from build123d import *

# Parameters (mm, degrees)
SKETCH_R          = 2.5
PAD_DEPTH         = 30
SKETCH001_R       = 4
PAD001_DEPTH      = 3
SKETCH002_R       = 1.5
POCKET_DEPTH      = 4.001
POCKET_DEPTH_BACK = -4.001


with BuildPart() as part:
    # Sketch → Pad (new body)
    with BuildSketch(Plane.XY):
        Circle(SKETCH_R)
    extrude(amount=PAD_DEPTH)

    # Sketch001 → Pad001 (join)
    with BuildSketch(Plane.XY):
        Circle(SKETCH001_R)
    extrude(amount=PAD001_DEPTH)

    # Sketch002 → Pocket (cut, two sides)
    with BuildSketch(Plane.XZ) as pocket_sk:
        with Locations((0, 27)):
            Circle(SKETCH002_R)
    extrude(amount=-POCKET_DEPTH, mode=Mode.SUBTRACT)
    extrude(pocket_sk.sketch, amount=-POCKET_DEPTH_BACK, mode=Mode.SUBTRACT)


solid = part.part
Here's how the part is built. I have some questions about the finished solid (model axes, mm). A direction names the side the tool comes from. Round coordinates to 2 decimals unless told otherwise and drop trailing zeros. Order: outer loops, then holes, each group sorted by start corner. A loop starts at its lowest first (then second) coordinate and runs counter-clockwise, first axis right, second up. Notation, with made-up numbers: (69.25, -16.5) -> (108.25, -16.5) arc R10 cw to (108.25, -2.5) -> close; hole circle Ø4 at (25, 19.25). An arc over 180 degrees is marked (long way). Return JSON: item names as keys, results as strings.
Q1. Which directions (+Z, -Z, +X, -X, +Y, -Y) give clear straight access to the entire face, cutting with the end or side of a thin tool? Please do faces 1 (the cylindrical face through (2.385, 0.751, 16.311)), 2 (the flat face through (0, 0, 30)).
Filled sheet:
{"face 1": "+Z", "face 2": "+Z, +X, -X, +Y, -Y"}
Q2. If we mould it in two halves opening along Z, with no side actions, what happens to faces 3 (the flat face through (0, 0, 0)), 4 (the cylindrical face through (-0.867, -3.905, 1.479)), 5 (the cylindrical face through (-1.5, -0.04, 27.07)), 6 (the flat face through (2, 2, 3))? For each: released by +Z, released by -Z, zero draft, split by the parting line, or undercut.
Filled sheet:
{"face 3": "released by -Z", "face 4": "zero draft", "face 5": "undercut", "face 6": "released by +Z"}
Q3. If we section it at D-D on z = 17: List the corners of the cut face in (x, y) for me, plus the area to 3 significant figures.
Filled sheet:
{"outline": "circle Ø5 at (0, 0)", "area": "19.6 mm^2"}
Q4. For pin 1 Ø1 at (y, z) = (2.5, 23) entering from +X; pin 2 Ø4 at (x, z) = (3, 13.5) entering from -Y; pin 3 Ø4 at (y, z) = (2, 20.5) entering from +X; pin 4 Ø2.5 at (x, z) = (0, 27) entering from +Y, each with a flat end and sliding along its axis, tell me the tip position at first contact or that it passes through.
Filled sheet:
{"pin 1": "stops at x = 1.5", "pin 2": "stops at y = -2.29", "pin 3": "stops at x = 2.5", "pin 4": "passes through"}
Q5. I need wall thicknesses on line 1 along Z through (x, y) = (0, -1.2); line 2 along Y through (x, z) = (2, 9.5); line 3 along Y through (x, z) = (0, 7). Which ranges of each line are inside material? Lowest first, please. Write a range as from..to.
Filled sheet:
{"line 1": "z = 0..25.5, 28.5..30", "line 2": "y = -1.5..1.5", "line 3": "y = -2.5..2.5"}
Q6. If we section it at A-A on x = 0: List the corners of the cut face in (y, z) for me.
Filled sheet:
{"outline": "(-4, 0) -> (4, 0) -> (4, 3) -> (2.5, 3) -> (2.5, 25.5) -> (-2.5, 25.5) -> (-2.5, 3) -> (-4, 3) -> close; (-2.5, 28.5) -> (2.5, 28.5) -> (2.5, 30) -> (-2.5, 30) -> close"}
Q7. If we section it at B-B on y = 0: List the corners of the cut face in (x, z) for me.
Filled sheet:
{"outline": "(-4, 0) -> (4, 0) -> (4, 3) -> (2.5, 3) -> (2.5, 30) -> (-2.5, 30) -> (-2.5, 3) -> (-4, 3) -> close; hole circle Ø3 at (0, 27)"}
Q8. If we section it at C-C on z = 27: List the corners of the cut face in (x, y) for me, plus the area to 3 significant figures.
Filled sheet:
{"outline": "(-1.5, -2) -> (-1.5, 2) arc R2.5 ccw to start; (1.5, -2) arc R2.5 ccw to (1.5, 2) -> close", "area": "5.59 mm^2"}
